from build123d import *

# Parameters (mm, degrees)
BOSS_EXTRUDE1_DEPTH = 25.4
FILLET1_R           = 5
FILLET2_R           = 5
FILLET3_R           = 5
SKETCH2_R           = 2.286
CUT_EXTRUDE2_DEPTH  = 81.112257119


with BuildPart() as part:
    # Sketch1 → Boss-Extrude1 (new body)
    with BuildSketch(Plane.XY):
        Polygon((0, 0), (5.147680359, -8.573294986), (44.26134523, -39.720064006), (63.5, -39.720064006), (63.5, -41.720064006), (43.562310597, -41.720064006), (3.619073412, -9.912694725), (-2, -0.554309869), (-10, -0.554309869), (-10, 20), (0, 20), align=None)
    extrude(amount=BOSS_EXTRUDE1_DEPTH)

    # Fillet1
    fillet1_edges = [part.edges().sort_by_distance(p)[0] for p in [
        (-2, -0.554309869, 12.7),
    ]]
    fillet(fillet1_edges, radius=FILLET1_R)

    # Fillet2
    fillet2_edges = [part.edges().sort_by_distance(p)[0] for p in [
        (0, 20, 12.7),
    ]]
    fillet(fillet2_edges, radius=FILLET2_R)

    # Fillet3
    fillet3_edges = [part.edges().sort_by_distance(p)[0] for p in [
        (-10, 20, 12.7),
    ]]
    fillet(fillet3_edges, radius=FILLET3_R - 0.0001)  # a hair under: the kernel refuses the full size

    # Sketch2 → Cut-Extrude2 (cut, through all)
    with BuildSketch(Plane.XY.offset(25.4)):
        with Locations((-4.829903584, 3.445690131)):
            Circle(SKETCH2_R)
    extrude(amount=-CUT_EXTRUDE2_DEPTH, mode=Mode.SUBTRACT)


solid = part.part
Can you work these out from the model? Positions are in its coordinate system, mm. A direction names the side the tool comes from. Coordinates: 2 decimals unless noted, no trailing zeros. Loops run counter-clockwise (first coordinate to the right, second up) from the corner with the lowest first, then second, coordinate; pieces in that order, holes last. Notation, with made-up numbers: (-16.5, 11.5) - (-0.5, 11.5) arc R24 cw to (-0.5, 32.5) - close; hole circle Ø6 at (45.5, 17.25). An arc over 180 degrees is marked (long way). Put each result on its own line as item: value. Start each with the question number.
Item 1: Suppose I cut it at C-C (x = 49). Please give me the cut outline in (y, z).
Item 2: Which directions (+Z, -Z, +X, -X, +Y, -Y) give clear straight access to the entire face, cutting with the end or side of a thin tool? Please do faces 1 (the face through (-7, -0.554, 13)), 2 (the face through (-8, 19, 13)).
Item 3: If I drill on line 1 along Y through (x, z) = (50, 22.5); line 2 along X through (y, z) = (7, 3.5); line 3 along X through (y, z) = (4, 24.75), over which ranges is the centre line in solid material (lowest first)?
Item 4: Suppose I cut it at D-D (y = -5.5). Please give me the cut outline in (x, z).
Item 5: For pin 1 (1.6 mm diameter, centred on x = -7.5, z = 16, fed in from -Y); pin 2 (1 mm diameter, centred on y = -27, z = 18, fed in from +X); pin 3 (10 mm diameter, centred on x = 56, z = 3, fed in from +Y); pin 4 (10 mm diameter, centred on x = 3, y = 8, fed in from +Z), each with a flat end and sliding along its axis, tell me the tip position at first contact or that it passes through.
Item 6: If we mould it in two halves opening along X, with no side actions, what happens to faces 3 (the face through (54, -39.72, 13)), 4 (the face through (-6.64, 2.05, 12.88)), 5 (the face through (0, 8, 13))? For each: +X half, -X half, draft (parallel to the pull), parting line (faces both ways), or undercut.
Item 7: Suppose I cut it at A-A (y = 4.5). Please give me the cut outline in (x, z), and give its area (3 significant figures).
Here are the results:
1. outline: (-41.72, 0) - (-39.72, 0) - (-39.72, 25.4) - (-41.72, 25.4) - close
2. face 1: +Z, -Z, -X, -Y
2. face 2: +Z, -Z, -X, +Y
3. line 1: -41.72 to -39.72
3. line 2: -10 to 0
3. line 3: -10 to -7.05, -2.61 to 0
4. outline: (0.97, 0) - (3.3, 0) - (3.3, 25.4) - (0.97, 25.4) - close
5. pin 1: y = -0.55
5. pin 2: x = 28.92
5. pin 3: y = -39.72
5. pin 4: z = 25.4
6. face 3: draft
6. face 4: undercut
6. face 5: +X half
7. outline: (-10, 0) - (-6.86, 0) - (-6.86, 25.4) - (-10, 25.4) - close; (-2.8, 0) - (0, 0) - (0, 25.4) - (-2.8, 25.4) - close
7. area: 151 mm²
